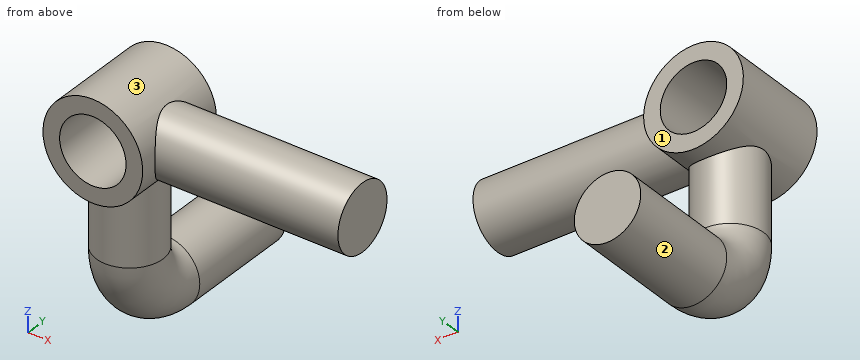
```python
from build123d import *

# Parameters (mm, degrees)
SKETCH1_R                = 1.5
SKETCH1_R_2              = 1
BOSS_EXTRUDE1_DEPTH      = 3
SKETCH3_R                = 1
BOSS_EXTRUDE4_REACH      = 7.895
SKETCH4_R                = 1
BOSS_EXTRUDE5_REACH      = 12.977
BOSS_EXTRUDE5_END_RADIUS = 1.5
SKETCH6_R                = 1


with BuildPart() as part:
    # Sketch1 → Boss-Extrude1 (new body)
    with BuildSketch(Plane(origin=(0, 0, 0), x_dir=(1, 0, 0), z_dir=(0, 1, 0))):
        with Locations(Location((0, 0, 0), (0, 0, 270))):
            Circle(SKETCH1_R)
        with Locations(Location((0, 0, 0), (0, 0, 270))):
            Circle(SKETCH1_R_2, mode=Mode.SUBTRACT)
    extrude(amount=-BOSS_EXTRUDE1_DEPTH)

    # Sketch4 → Boss-Extrude4 (add, up to next)
    with BuildSketch(Plane.XY.offset(-1.5), mode=Mode.PRIVATE) as boss_extrude4_sk1:
        with Locations(Location((0, -1.5, 0), (0, 0, 180))):
            Circle(SKETCH4_R)
    boss_extrude4_tool1 = extrude(boss_extrude4_sk1.sketch, amount=BOSS_EXTRUDE4_REACH, mode=Mode.PRIVATE) - part.part


with BuildPart() as body_2:
    # Sweep1: sweep along a path in Sketch2
    with BuildLine(Plane(origin=(0, 0, 0), x_dir=(0, 0, -1), z_dir=(1, 0, 0))) as sweep1_path:
        Line((1.5, -1.5), (3.5, -1.5))
        ThreePointArc((3.5, -1.5), (4.560660172, -1.060660172), (5, 0))
        Line((5, 0), (5, 3.5))
    # Sketch3 → Sweep1 (sweep)
    with BuildSketch(Plane(origin=(0, 3.5, 0), x_dir=(1, 0, 0), z_dir=(0, 1, 0))):
        with Locations((0, 5)):
            Circle(SKETCH3_R)
    sweep(path=sweep1_path.line)


with BuildPart() as part_1:
    add(part.part)

    add(body_2.part)  # Boss-Extrude4 merges body 2
    add(boss_extrude4_tool1.solids().sort_by_distance((0, -1.5, -1.5))[0])
    add(boss_extrude4_tool1.solids().sort_by_distance((0, -1.5, -1.5))[1])

    # Boss-Extrude5: up to this cylinder (the profile starts outside it)
    boss_extrude5_end = Plane(origin=(0, -1.5, 0), z_dir=(0, 1, 0)) * Cylinder(BOSS_EXTRUDE5_END_RADIUS, 29.954, mode=Mode.PRIVATE)
    # Sketch6 → Boss-Extrude5 (add, up to the surface)
    with BuildSketch(Plane(origin=(7, 0, 0), x_dir=(0, 0, -1), z_dir=(1, 0, 0)), mode=Mode.PRIVATE) as boss_extrude5_sk1:
        with Locations((0, -1.5)):
            Circle(SKETCH6_R)
    boss_extrude5_tool1 = extrude(boss_extrude5_sk1.sketch, amount=-BOSS_EXTRUDE5_REACH, mode=Mode.PRIVATE) - boss_extrude5_end
    add(boss_extrude5_tool1.solids().sort_by_distance((7, -1.5, 0))[0])


solid = part_1.part
```
Here's how the part is built. I have some questions about the finished solid (model axes, mm). Face numbers are marked on the shaded views. A direction names the side the tool comes from. Round coordinates to 2 decimals unless told otherwise and drop trailing zeros. Order: outer loops, then holes, each group sorted by start corner. A loop starts at its lowest first (then second) coordinate and runs counter-clockwise, first axis right, second up. Notation, with made-up numbers: (13.25, 49.5) -> (64.25, 49.5) arc R36 cw to (64.25, 85.5) -> close; hole circle Ø11 at (72, 0.25). An arc over 180 degrees is marked (long way). Use a Markdown table: item, result. Add a question column.
(1) For the marked faces 1, 2 and 3, which set-ups out of +Z, -Z, +X, -X, +Y, -Y let a thin tool reach every point of the face, with its end or its side?
(2) Suppose I cut it at B-B, the plane x = 0. Please give me the cut outline in (y, z).
(3) Suppose I cut it at C-C, the plane x = 1.25. Please give me the cut outline in (y, z), and give its area (3 significant figures).
(4) For pin 1 Ø3 at (y, z) = (-2, -3) entering from -X; pin 2 Ø2 at (x, z) = (4.5, -1) entering from +Y; pin 3 Ø4 at (x, z) = (5, 0) entering from -Y, each with a flat end and sliding along its axis, tell me the tip position at first contact or that it passes through.
(5) Suppose I cut it at D-D, the plane z = -3.25. Please give me the cut outline in (x, y), and give its area (3 significant figures).
(6) I need wall thicknesses on line 1 along X through (y, z) = (-2.05, 0); line 2 along Z through (x, y) = (0.25, -0.75); line 3 along X through (y, z) = (2.5, -4.5). Which ranges of each line are inside material? Lowest first, please.
(7) Suppose I cut it at A-A, the plane z = 0. Please give me the cut outline in (x, y), and give its area (3 significant figures).
Verdict:
| question | item | result |
|---|---|---|
| 1 | face 1 | +Z, +X, -X, +Y |
| 1 | face 2 | +Y |
| 1 | face 3 | none |
| 2 | outline | (-3, -1.5) -> (-2.5, -1.5) -> (-2.5, -3.5) arc R2.5 ccw to (0, -6) -> (3.5, -6) -> (3.5, -4) -> (0, -4) arc R0.5 cw to (-0.5, -3.5) -> (-0.5, -1.5) -> (0, -1.5) -> (0, -1) -> (-3, -1) -> close; (-3, 1) -> (0, 1) -> (0, 1.5) -> (-3, 1.5) -> close |
| 3 | outline | (-3, -0.83) -> (-2.06, -0.83) arc R1 ccw to (-0.94, -0.83) -> (0, -0.83) -> (0, 0.83) -> (-0.94, 0.83) arc R1 ccw to (-2.06, 0.83) -> (-3, 0.83) -> close |
| 3 | area | 5.23 mm2 |
| 4 | pin 1 | x = -1 |
| 4 | pin 2 | y = -0.5 |
| 4 | pin 3 | y = -2.5 |
| 5 | outline | circle Ø2 at (0, -1.5) |
| 5 | area | 3.14 mm2 |
| 6 | line 1 | -1.5 to -1, 1 to 7 |
| 6 | line 2 | -5.85 to -0.97, 0.97 to 1.48 |
| 6 | line 3 | -0.87 to 0.87 |
| 7 | outline | (-1.5, -3) -> (-1, -3) -> (-1, 0) -> (-1.5, 0) -> close; (1, -3) -> (1.5, -3) -> (1.5, -2.5) -> (7, -2.5) -> (7, -0.5) -> (1.5, -0.5) -> (1.5, 0) -> (1, 0) -> close |
| 7 | area | 14.0 mm2 |
